from build123d import *

# Parameters (mm, degrees)
BOSS_EXTRUDE1_DEPTH   = 38
BOSS_EXTRUDE1_2_DEPTH = 38
SKETCH2_W             = 42.5
SKETCH2_H             = 5.7
BOSS_EXTRUDE2_DEPTH   = 2
BOSS_EXTRUDE3_DEPTH   = 18
SKETCH4_W             = 42.5
SKETCH4_H             = 40
BOSS_EXTRUDE4_DEPTH   = 2
SKETCH5_W             = 37.1
SKETCH5_H             = 11.85
CUT_EXTRUDE1_DEPTH    = 81.281509747


with BuildPart() as part:
    # Sketch1 → Boss-Extrude1 (new body)
    with BuildSketch(Plane(origin=(0, 0, 0), x_dir=(1, 0, 0), z_dir=(0, 1, 0))):
        Polygon((-62.898983402, -26.09346473), (-62.898983402, -24.39346473), (-62.198983402, -24.39346473), (-62.198983402, -22.39346473), (-64.898983402, -22.39346473), (-64.898983402, -28.09346473), (-62.198983402, -28.09346473), (-62.198983402, -26.09346473), align=None)
    extrude(amount=BOSS_EXTRUDE1_DEPTH)



with BuildPart() as body_2:
    # Sketch1 → Boss-Extrude1 2 (new body)
    with BuildSketch(Plane(origin=(0, 0, 0), x_dir=(1, 0, 0), z_dir=(0, 1, 0))):
        Polygon((-25.098983402, -22.39346473), (-25.098983402, -24.39346473), (-24.398983402, -24.39346473), (-24.398983402, -26.09346473), (-25.098983402, -26.09346473), (-25.098983402, -28.09346473), (-22.398983402, -28.09346473), (-22.398983402, -22.39346473), align=None)
    extrude(amount=BOSS_EXTRUDE1_2_DEPTH)


with BuildPart() as part_1:
    add(part.part)

    add(body_2.part)  # Boss-Extrude2 merges body 2
    # Sketch2 → Boss-Extrude2 (add)
    with BuildSketch(Plane(origin=(0, 0, 0), x_dir=(1, 0, 0), z_dir=(0, 1, 0))):
        with Locations((-43.648983402, -25.24346473)):
            Rectangle(SKETCH2_W, SKETCH2_H)
    extrude(amount=-BOSS_EXTRUDE2_DEPTH)

    # Sketch3 → Boss-Extrude3 (add)
    with BuildSketch(Plane(origin=(0, 0, 22.39346473), x_dir=(-1, 0, 0), z_dir=(0, 0, -1))):
        Polygon((64.898983402, 38), (62.198983402, 38), (62.198983402, 0), (25.098983402, 0), (25.098983402, 38), (22.398983402, 38), (22.398983402, -2), (64.898983402, -2), align=None)
    extrude(amount=BOSS_EXTRUDE3_DEPTH)

    # Sketch4 → Boss-Extrude4 (add)
    with BuildSketch(Plane(origin=(0, 0, 4.39346473), x_dir=(-1, 0, 0), z_dir=(0, 0, -1))):
        with Locations((43.648983402, 18)):
            Rectangle(SKETCH4_W, SKETCH4_H)
    extrude(amount=BOSS_EXTRUDE4_DEPTH)

    # Sketch5 → Cut-Extrude1 (cut, through all)
    with BuildSketch(Plane(origin=(0, 0, 0), x_dir=(1, 0, 0), z_dir=(0, 1, 0))):
        with Locations((-43.648983402, -10.31846473)):
            Rectangle(SKETCH5_W, SKETCH5_H)
    extrude(amount=-CUT_EXTRUDE1_DEPTH, mode=Mode.SUBTRACT)


solid = part_1.part
Design review of the part built by this model. Coordinates are the model's own, in mm. A direction names the side the tool comes from. Give positions to 0.01 mm unless a question says otherwise; leave off trailing zeros. Loops run counter-clockwise (first coordinate to the right, second up) from the corner with the lowest first, then second, coordinate; pieces in that order, holes last. Notation, with made-up numbers: M -39,-4.5 L -10,-4.5 A20 cw -10,32.5 Z; hole C 7.5,72 d3. An arc over 180 degrees is marked long. Answer as a JSON object with one key per item and string values.
Item 1: We need section A-A (z = 9.75). State the section outline as (x, y) points, and give its area (3 significant figures).
Output values:
{"outline": "M -64.9,-2 L -62.2,-2 L -62.2,38 L -64.9,38 Z; M -25.1,-2 L -22.4,-2 L -22.4,38 L -25.1,38 Z", "area": "216 mm2"}
Item 2: We need section B-B (x = -35). State the section outline as (y, z) points.
Output values:
{"outline": "M -2,2.39 L 38,2.39 L 38,4.39 L -2,4.39 Z; M -2,16.24 L 0,16.24 L 0,28.09 L -2,28.09 Z"}
Item 3: Mouldability with a two-part tool opening along Z and no side actions: class faces 1 (the face through (-44, 38, 4)), 2 (the face through (-43, 18, 2.393)), 3 (the face through (-24.399, 19, 25)) as pulls with the +Z half, pulls with the -Z half, needs draft (parallel to the pull), parting line crosses it, or undercut.
Output values:
{"face 1": "needs draft", "face 2": "pulls with the -Z half", "face 3": "undercut"}
Item 4: For P1, Ø3.5, axis at x = -46, z = 24, coming from the +Y side; P2, Ø18.5, axis at x = -41.5, y = 27, coming from the +Z side, all flat-tipped, find the tip position at first contact; note any pin that passes through.
Output values:
{"P1": "stops at y = 0", "P2": "stops at z = 4.39"}
Item 5: Machinability: for faces 4 (the face through (-62.199, 19, 27)), 5 (the face through (-22.399, 18, 15)), 6 (the face through (-62.899, 19, 25)), 7 (the face through (-44, -1, 16.243)), which of the approach directions +Z, -Z, +X, -X, +Y, -Y give a long, thin tool a straight path to every point of the face, cutting with its end or side? Answer none if there is none.
Output values:
{"face 4": "+Z, +Y", "face 5": "+Z, -Z, +X, +Y, -Y", "face 6": "+Y", "face 7": "+Y, -Y"}
Item 6: We need section C-C (y = 7). State the section outline as (x, z) points, and give its area (3 significant figures).
Output values:
{"outline": "M -64.9,2.39 L -22.4,2.39 L -22.4,28.09 L -25.1,28.09 L -25.1,26.09 L -24.4,26.09 L -24.4,24.39 L -25.1,24.39 L -25.1,4.39 L -62.2,4.39 L -62.2,24.39 L -62.9,24.39 L -62.9,26.09 L -62.2,26.09 L -62.2,28.09 L -64.9,28.09 Z", "area": "211 mm2"}
Item 7: Wall thickness on line 1 along X through (y, z) = (9, 5.5); line 2 along Z through (x, y) = (-24.5, 34); line 3 along Z through (x, y) = (-47.5, 30.5): over which ranges is each line inside the solid? List them lowest first.
Output values:
{"line 1": "x = -64.9 to -62.2, -25.1 to -22.4", "line 2": "z = 2.39 to 24.39, 26.09 to 28.09", "line 3": "z = 2.39 to 4.39"}
